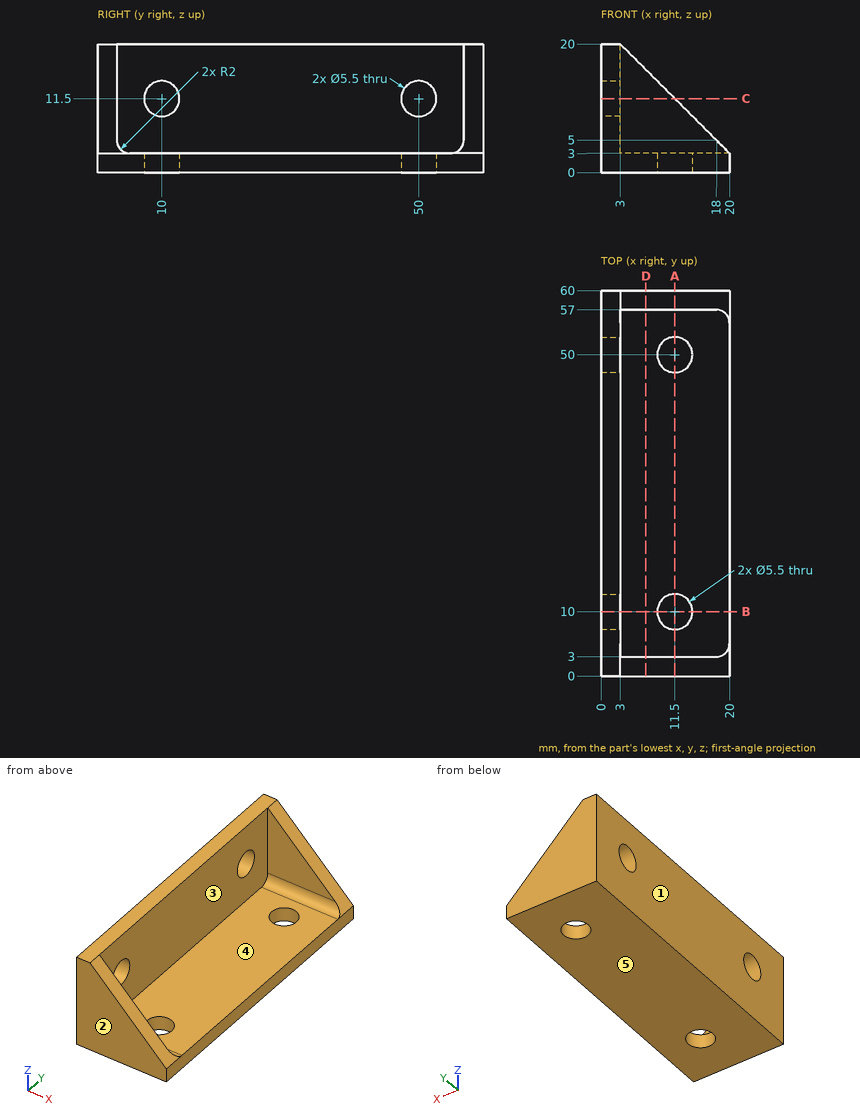
The figure shows three views and two pictorial views of one solid part (mm, origin at its lowest corner). Answer the questions. A direction names the side the tool comes from. Give positions to 0.01 mm unless a question says otherwise; leave off trailing zeros. Write each loop counter-clockwise with the first axis right and the second up, starting at its lowest first coordinate (ties: lowest second). Pieces come first, ordered by that corner, then holes. Notation, with made-up numbers: (47, 16) -> (61, 16) arc R22 cw to (61, 26) -> close; hole circle Ø4 at (26.5, 63.25). An arc over 180 degrees is marked (long way). Write each question's results on one line, items separated by ' | '.
1. A tool of negligible diameter and unlimited length cuts with its end or side. For the marked faces 4 and 5, from which of +Z, -Z, +X, -X, +Y, -Y can it reach the whole face along a straight path? Write none if from no direction.
Data:
face 4: +Z, +X | face 5: -Z, +X, -X, +Y, -Y
2. Each of these flat-tipped pins is pushed along its axis until it touches: pin 1 Ø5 at (x, y) = (13, 37) entering from +Z; pin 2 Ø5 at (x, y) = (11.5, 10) entering from -Z; pin 3 Ø5 at (y, z) = (17, 10.5) entering from +X. Where does it stop, or does it pass through?
Data:
pin 1: z = 3 | pin 2: through | pin 3: x = 3
3. Find section D-D on x = 7. Determine the outline of the cut face in (y, z), and give its area (3 significant figures).
Data:
outline: (0, 0) -> (60, 0) -> (60, 16) -> (57, 16) -> (57, 5) arc R2 cw to (55, 3) -> (5, 3) arc R2 cw to (3, 5) -> (3, 16) -> (0, 16) -> close | area: 260 mm^2
4. Find section B-B on y = 10. Determine the outline of the cut face in (x, z).
Data:
outline: (0, 0) -> (8.75, 0) -> (8.75, 3) -> (3, 3) -> (3, 8.75) -> (0, 8.75) -> close; (0, 14.25) -> (3, 14.25) -> (3, 20) -> (0, 20) -> close; (14.25, 0) -> (20, 0) -> (20, 3) -> (14.25, 3) -> close
5. Straight lines are drawn through the part: L1, parallel to Y at x = 11.5, z = 0.65; L2, parallel to Y at x = 12.25, z = 7.75; L3, parallel to Y at x = 13.5, z = 2. For each, find the intervals that lie inside material, in ascending order.
Data:
L1: 0 to 7.25, 12.75 to 47.25, 52.75 to 60 | L2: 0 to 3, 57 to 60 | L3: 0 to 8.11, 11.89 to 48.11, 51.89 to 60
6. Find section C-C on z = 11.5. Determine the outline of the cut face in (x, y).
Data:
outline: (0, 0) -> (11.5, 0) -> (11.5, 3) -> (3, 3) -> (3, 7.25) -> (0, 7.25) -> close; (0, 12.75) -> (3, 12.75) -> (3, 47.25) -> (0, 47.25) -> close; (0, 52.75) -> (3, 52.75) -> (3, 57) -> (11.5, 57) -> (11.5, 60) -> (0, 60) -> close
7. Find section A-A on x = 11.5. Determine the outline of the cut face in (y, z).
Data:
outline: (0, 0) -> (7.25, 0) -> (7.25, 3) -> (5, 3) arc R2 cw to (3, 5) -> (3, 11.5) -> (0, 11.5) -> close; (12.75, 0) -> (47.25, 0) -> (47.25, 3) -> (12.75, 3) -> close; (52.75, 0) -> (60, 0) -> (60, 11.5) -> (57, 11.5) -> (57, 5) arc R2 cw to (55, 3) -> (52.75, 3) -> close
8. Determine the mould class of the marked faces 1, 2 and 3 for opening direction Y: +Y half, -Y half, draft (parallel to the pull), parting line (faces both ways), or undercut.
Data:
face 1: draft | face 2: -Y half | face 3: undercut
